```python
from build123d import *

# Parameters (mm, degrees)
SKETCH_1_W          = 182
SKETCH_1_H          = 50
SKETCH_1_R          = 2
EXTRUDE_1_DEPTH     = 2
SKETCH_2_R          = 1.6
CUT_EXTRUDE_1_DEPTH = 95.392796335
SKETCH_3_W          = 43
SKETCH_3_H          = 34
SKETCH_3_W_2        = 42.5
SKETCH_3_H_2        = 30
CUT_EXTRUDE_2_DEPTH = 95.392796335


with BuildPart() as part:
    # 草图1 → 凸台-拉伸1 (new body)
    with BuildSketch(Plane.XY):
        Rectangle(SKETCH_1_W, SKETCH_1_H)
        with Locations((-86, 15)):
            Circle(SKETCH_1_R, mode=Mode.SUBTRACT)
        with Locations((86, 15)):
            Circle(SKETCH_1_R, mode=Mode.SUBTRACT)
        with Locations((-86, -15)):
            Circle(SKETCH_1_R, mode=Mode.SUBTRACT)
        with Locations((86, -15)):
            Circle(SKETCH_1_R, mode=Mode.SUBTRACT)
    extrude(amount=EXTRUDE_1_DEPTH)

    # 草图2 → 切除-拉伸1 (cut, through all)
    with BuildSketch(Plane.XY.offset(2)):
        with Locations((-27.5, 8.5)):
            Circle(SKETCH_2_R)
        with Locations((-27.5, -8.5)):
            Circle(SKETCH_2_R)
        with Locations((27.5, 8.5)):
            Circle(SKETCH_2_R)
        with Locations((27.5, -8.5)):
            Circle(SKETCH_2_R)
    extrude(amount=-CUT_EXTRUDE_1_DEPTH, mode=Mode.SUBTRACT)

    # 草图3 → 切除-拉伸2 (cut, through all)
    with BuildSketch(Plane.XY.offset(2)):
        Rectangle(SKETCH_3_W, SKETCH_3_H)
        with Locations((-54.75, 0)):
            Rectangle(SKETCH_3_W_2, SKETCH_3_H_2)
        with Locations((54.75, 0)):
            Rectangle(SKETCH_3_W_2, SKETCH_3_H_2)
    extrude(amount=-CUT_EXTRUDE_2_DEPTH, mode=Mode.SUBTRACT)


solid = part.part
```
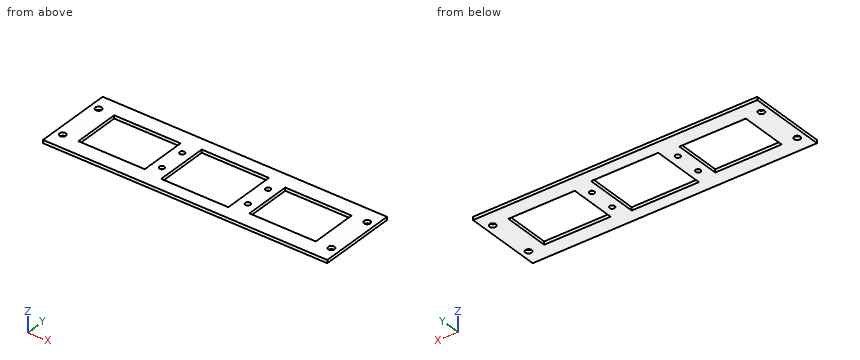
Can you work these out from the model? Positions are in its coordinate system, mm. Round coordinates to 2 decimals unless told otherwise and drop trailing zeros. Loops run counter-clockwise (first coordinate to the right, second up) from the corner with the lowest first, then second, coordinate; pieces in that order, holes last.
Item 1: Suppose I cut it at D-D, the plane x = -55. Write out the boundary of the cut face in (y, z), then the cut area to 3 significant figures.
Item 2: Suppose I cut it at C-C, the plane y = -8.5. Write out the boundary of the cut face in (x, z).
Item 3: Suppose I cut it at A-A, the plane x = -86. Write out the boundary of the cut face in (y, z).
Item 4: Suppose I cut it at B-B, the plane y = -0.5. Write out the boundary of the cut face in (x, z), then the cut area to 3 significant figures.
Item 5: Please list where these lines run through material, in increasing order: L1, parallel to X at y = 6, z = 0.7; L2, parallel to Y at x = -27.5, z = 1.1; L3, parallel to Y at x = 86, z = 1.
Reported:
1. outline: (-25, 0) - (-15, 0) - (-15, 2) - (-25, 2) - close; (15, 0) - (25, 0) - (25, 2) - (15, 2) - close
1. area: 40.0 mm2
2. outline: (-91, 0) - (-76, 0) - (-76, 2) - (-91, 2) - close; (-33.5, 0) - (-29.1, 0) - (-29.1, 2) - (-33.5, 2) - close; (-25.9, 0) - (-21.5, 0) - (-21.5, 2) - (-25.9, 2) - close; (21.5, 0) - (25.9, 0) - (25.9, 2) - (21.5, 2) - close; (29.1, 0) - (33.5, 0) - (33.5, 2) - (29.1, 2) - close; (76, 0) - (91, 0) - (91, 2) - (76, 2) - close
3. outline: (-25, 0) - (-17, 0) - (-17, 2) - (-25, 2) - close; (-13, 0) - (13, 0) - (13, 2) - (-13, 2) - close; (17, 0) - (25, 0) - (25, 2) - (17, 2) - close
4. outline: (-91, 0) - (-76, 0) - (-76, 2) - (-91, 2) - close; (-33.5, 0) - (-21.5, 0) - (-21.5, 2) - (-33.5, 2) - close; (21.5, 0) - (33.5, 0) - (33.5, 2) - (21.5, 2) - close; (76, 0) - (91, 0) - (91, 2) - (76, 2) - close
4. area: 108 mm2
5. L1: x = -91 to -76, -33.5 to -21.5, 21.5 to 33.5, 76 to 91
5. L2: y = -25 to -10.1, -6.9 to 6.9, 10.1 to 25
5. L3: y = -25 to -17, -13 to 13, 17 to 25
